The model under review builds one solid part; all positions refer to its coordinate system, in mm. Face numbers are marked on the shaded views. A direction names the side the tool comes from. Round coordinates to 2 decimals unless told otherwise and drop trailing zeros. Order: outer loops, then holes, each group sorted by start corner. A loop starts at its lowest first (then second) coordinate and runs counter-clockwise, first axis right, second up. Notation, with made-up numbers: M 66.25,36 L 92.25,36 A3 cw 92.25,40 Z; hole C -36,63.5 d4. An arc over 180 degrees is marked long. Answer as a JSON object with one key per item and string values. Group by question number.
1) To check wall thickness, follow line 1 (X direction, y = -98, z = 49.5); line 2 (Z direction, x = 0, y = -11.75); line 3 (X direction, y = -9, z = -161). State the ranges of each line that lie inside material, in increasing order.
2) Consider section B-B, the plane y = -12.5. Count the separate pieces of the cut face and the enclosed holes in it, then the cut area to 3 significant figures.
3) The part is to be moulded in two halves that separate along X. For the marked faces 4 and 5, say which applies: +X half, -X half, draft (parallel to the pull), parting line (faces both ways), or undercut.
4) Consider section C-C, the plane x = 0. Write out the cut boundary in (y, z).
5) Insertion check: pin 1 Ø7.5 at (y, z) = (-6.5, 33.5) entering from -X; pin 2 Ø9.5 at (x, y) = (3.5, -13.5) entering from -Z; pin 3 Ø8 at (x, y) = (-200, -22.5) entering from -Z. Each pin has a flat end and moves straight along its axis. Give the tip position at first contact, or say it passes through.
6) Consider section A-A, the plane z = 0. Write out the cut boundary in (x, y), then the cut area to 3 significant figures.
7) For the marked faces 1, 2 and 3, list the 3-axis set-ups (+Z, -Z, +X, -X, +Y, -Y) from which the entire face can be reached by the end or side of a thin tool; tool diameter is ignored.
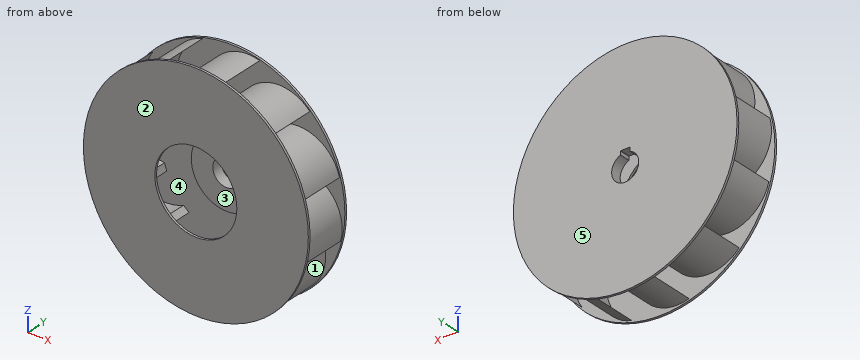
```python
from build123d import *

# Parameters (mm, degrees)
SKETCH_R           = 251.288776
PAD_DEPTH          = 5
SKETCH001_R        = 78.787228
PAD001_DEPTH       = 19
POCKET_DEPTH       = 24.001
PAD002_DEPTH       = 100
POLARPATTERN_COUNT = 12
SKETCH004_R        = 252.739118
PAD003_DEPTH       = 5
SKETCH005_R        = 92.174815
POCKET001_DEPTH    = 5


with BuildPart() as part:
    # Sketch → Pad (new body)
    with BuildSketch(Plane.XZ):
        Circle(SKETCH_R)
    extrude(amount=PAD_DEPTH)

    # Sketch001 (on Face3 of Pad) → Pad001 (join)
    with BuildSketch(Plane.XZ.offset(5)):
        Circle(SKETCH001_R)
    extrude(amount=PAD001_DEPTH)

    # Sketch002 (on Face5 of Pad001) → Pocket (cut, through all)
    with BuildSketch(Plane.XZ.offset(24)):
        with BuildLine():
            ThreePointArc((-11.342065, 28.248508), (0.09221, -30.440304), (11.170717, 28.316704))
            ThreePointArc((10.466113, 29.352113), (10.658972, 28.725907), (11.170717, 28.316704))
            Line((10.466113, 29.352113), (10.466113, 36.343864))
            ThreePointArc((10.466113, 36.343864), (10.16761, 37.064515), (9.446959, 37.363018))
            Line((9.446959, 37.363018), (-9.589921, 37.363018))
            ThreePointArc((-9.589921, 37.363018), (-10.209482, 37.106387), (-10.466113, 36.486826))
            Line((-10.466113, 36.486826), (-10.466113, 29.544133))
            ThreePointArc((-11.342065, 28.248508), (-10.705649, 28.762158), (-10.466113, 29.544133))
        make_face()
    extrude(amount=-POCKET_DEPTH, mode=Mode.SUBTRACT)

    # Sketch003 (on Face3 of Pocket) → Pad002 (join)
    with BuildSketch(Plane.XZ.offset(5)):
        with BuildLine():
            ThreePointArc((-44.856391, 154.010557), (-52.493731, 151.577556), (-60, 148.766083))
            ThreePointArc((60, 241.615551), (-23.506563, 225.571041), (-60, 148.766083))
            ThreePointArc((60, 241.615551), (-10.953355, 219.986234), (-44.856391, 154.010557))
        make_face()
    pad002 = extrude(amount=PAD002_DEPTH)

    # PolarPattern: Pad002 ×12 about axis
    polarpattern_axis = Axis((0, -5, 0), (0, -1, 0))
    for i in range(1, POLARPATTERN_COUNT):
        add(pad002.rotate(polarpattern_axis, i * 360 / POLARPATTERN_COUNT))

    # Sketch004 (on Face55 of PolarPattern) → Pad003 (join)
    with BuildSketch(Plane.XZ.offset(105)):
        Circle(SKETCH004_R)
    extrude(amount=PAD003_DEPTH)

    # Sketch005 (on Face3 of Pad003) → Pocket001 (cut)
    with BuildSketch(Plane.XZ.offset(110)):
        Circle(SKETCH005_R)
    extrude(amount=-POCKET001_DEPTH, mode=Mode.SUBTRACT)


solid = part.part
```
Results list:
{
 "1": {"line 1": "-243.98 to -242.13, -189.79 to -169.5, 152.58 to 194.39", "line 2": "-238.86 to -227.89, -78.79 to -30.44, 37.36 to 78.79, 227.89 to 238.86", "line 3": "-41.96 to -23.64, 44.07 to 59.51, 124.89 to 139.25, 186.54 to 189.55"},
 "2": {"separate pieces": "13", "enclosed holes": "1", "area": "37,300 mm^2"},
 "3": {"face 4": "undercut", "face 5": "draft"},
 "4": {"outline": "M -110,-252.74 L -105,-252.74 L -105,-238.86 L -5,-238.86 L -5,-251.29 L 0,-251.29 L 0,-30.44 L -24,-30.44 L -24,-78.79 L -5,-78.79 L -5,-227.89 L -105,-227.89 L -105,-92.17 L -110,-92.17 Z; M -110,92.17 L -105,92.17 L -105,227.89 L -5,227.89 L -5,78.79 L -24,78.79 L -24,37.36 L 0,37.36 L 0,251.29 L -5,251.29 L -5,238.86 L -105,238.86 L -105,252.74 L -110,252.74 Z"},
 "5": {"pin 1": "x = -249.48", "pin 2": "z = -239.34", "pin 3": "z = -126.96"},
 "6": {"outline": "M -252.74,-110 L -92.17,-110 L -92.17,-105 L -227.89,-105 L -227.89,-5 L -78.79,-5 L -78.79,-24 L -30.44,-24 L -30.44,0 L -251.29,0 L -251.29,-5 L -238.86,-5 L -238.86,-105 L -252.74,-105 Z; M 30.44,-24 L 78.79,-24 L 78.79,-5 L 227.89,-5 L 227.89,-105 L 92.17,-105 L 92.17,-110 L 252.74,-110 L 252.74,-105 L 238.86,-105 L 238.86,-5 L 251.29,-5 L 251.29,0 L 30.44,0 Z", "area": "7,850 mm^2"},
 "7": {"face 1": "none", "face 2": "+Z, -Z, +X, -X, -Y", "face 3": "-Y"}
}
